from build123d import *

# Parameters (mm, degrees)
SKIZZE1_W                       = 89.6
SKIZZE1_H                       = 46
SKIZZE1_W_2                     = 86
SKIZZE1_H_2                     = 43
AUFSATZ_LINEAR_AUSTRAGEN1_DEPTH = 1
SKIZZE1_3_W                     = 89.6
SKIZZE1_3_H                     = 46
SKIZZE1_3_W_2                   = 86
SKIZZE1_3_H_2                   = 43
AUFSATZ_LINEAR_AUSTRAGEN2_DEPTH = 50
SKIZZE2_W                       = 5.5
SKIZZE2_H                       = 5.5
SKIZZE2_R                       = 1.45
AUFSATZ_LINEAR_AUSTRAGEN3_DEPTH = 15
SKIZZE3_W                       = 5.5
SKIZZE3_H                       = 5.5
AUFSATZ_LINEAR_AUSTRAGEN4_DEPTH = 0.5
FASE1_SIZE                      = 5.5
SKIZZE4_W                       = 4.158916141
SKIZZE4_H                       = 8.076735696
SCHNITT_LINEAR_AUSTRAGEN1_DEPTH = 10
SKIZZE5_W                       = 22.047742135
SKIZZE5_H                       = 8.787632461
SCHNITT_LINEAR_AUSTRAGEN2_DEPTH = 10
SKIZZE6_W                       = 19.779455906
SKIZZE6_H                       = 6.441932887
SCHNITT_LINEAR_AUSTRAGEN3_DEPTH = 10
SKIZZE9_W                       = 20
SKIZZE9_H                       = 6
AUFSATZ_LINEAR_AUSTRAGEN6_DEPTH = 10
SKIZZE10_R                      = 2.25
SCHNITT_LINEAR_AUSTRAGEN5_DEPTH = 10
SKIZZE11_W                      = 75
SKIZZE11_H                      = 0.1
SCHNITT_LINEAR_AUSTRAGEN6_DEPTH = 37.646803
SKIZZE12_W                      = 12
SKIZZE12_H                      = 4
AUFSATZ_LINEAR_AUSTRAGEN7_DEPTH = 20
SCHNITT_LINEAR_AUSTRAGEN7_REACH = 88.161
SKIZZE13_R                      = 2.25
SKIZZE14_R                      = 3.7
SCHNITT_LINEAR_AUSTRAGEN8_DEPTH = 2
SKIZZE15_W                      = 89.6
SKIZZE15_H                      = 4.2
AUFSATZ_LINEAR_AUSTRAGEN8_DEPTH = 20
FASE2_SIZE                      = 4.5
FASE3_SIZE                      = 5
FASE4_SIZE                      = 5
FASE5_SIZE                      = 6


# Some blends are built 0.0001 mm under size
with BuildPart() as part:
    # Skizze1 → Aufsatz-Linear austragen1 (new body)
    # profile 1 of 2: a face of its own
    with BuildSketch(Plane.XY):
        with Locations((0, -0.3)):
            Rectangle(SKIZZE1_W, SKIZZE1_H)
        Rectangle(SKIZZE1_W_2, SKIZZE1_H_2, mode=Mode.SUBTRACT)
    # profile 2 of 2: a face of its own
    with BuildSketch(Plane.XY):
        Rectangle(SKIZZE1_W_2, SKIZZE1_H_2)
    extrude(amount=AUFSATZ_LINEAR_AUSTRAGEN1_DEPTH)

    # Skizze1<3> → Aufsatz-Linear austragen2 (add)
    with BuildSketch(Plane.XY):
        with Locations((0, -0.3)):
            Rectangle(SKIZZE1_3_W, SKIZZE1_3_H)
        Rectangle(SKIZZE1_3_W_2, SKIZZE1_3_H_2, mode=Mode.SUBTRACT)
    extrude(amount=AUFSATZ_LINEAR_AUSTRAGEN2_DEPTH)

    # Skizze2 → Aufsatz-Linear austragen3 (add)
    # profile 1 of 4: a face of its own
    with BuildSketch(Plane.XY.offset(50)):
        with Locations((-40.25, 18.75)):
            Rectangle(SKIZZE2_W, SKIZZE2_H)
        with Locations((-40.5, 19)):
            Circle(SKIZZE2_R, mode=Mode.SUBTRACT)
    # profile 2 of 4: a face of its own
    with BuildSketch(Plane.XY.offset(50)):
        with Locations((-40.25, -18.75)):
            Rectangle(SKIZZE2_W, SKIZZE2_H)
        with Locations(Location((-40.5, -19, 0), (0, 0, 180))):
            Circle(SKIZZE2_R, mode=Mode.SUBTRACT)
    # profile 3 of 4: a face of its own
    with BuildSketch(Plane.XY.offset(50)):
        with Locations((40.25, -18.75)):
            Rectangle(SKIZZE2_W, SKIZZE2_H)
        with Locations((40.5, -19)):
            Circle(SKIZZE2_R, mode=Mode.SUBTRACT)
    # profile 4 of 4: a face of its own
    with BuildSketch(Plane.XY.offset(50)):
        with Locations((40.25, 18.75)):
            Rectangle(SKIZZE2_W, SKIZZE2_H)
        with Locations(Location((40.5, 19, 0), (0, 0, 180))):
            Circle(SKIZZE2_R, mode=Mode.SUBTRACT)
    extrude(amount=-AUFSATZ_LINEAR_AUSTRAGEN3_DEPTH)

    # Skizze3 → Aufsatz-Linear austragen4 (add)
    with BuildSketch(Plane(origin=(0, 0, 35), x_dir=(-1, 0, 0), z_dir=(0, 0, -1))):
        with Locations((-40.25, 18.75)):
            Rectangle(SKIZZE3_W, SKIZZE3_H)
        with Locations((-40.25, -18.75)):
            Rectangle(SKIZZE3_W, SKIZZE3_H)
        with Locations((40.25, -18.75)):
            Rectangle(SKIZZE3_W, SKIZZE3_H)
        with Locations((40.25, 18.75)):
            Rectangle(SKIZZE3_W, SKIZZE3_H)
    extrude(amount=AUFSATZ_LINEAR_AUSTRAGEN4_DEPTH)

    # Fase1
    fase1_edges = [part.edges().sort_by_distance(p)[0] for p in [
        (43, 18.75, 34.5),
        (40.25, 21.5, 34.5),
        (-40.25, -21.5, 34.5),
        (-43, -18.75, 34.5),
        (-43, 18.75, 34.5),
        (-40.25, 21.5, 34.5),
        (40.25, -21.5, 34.5),
        (43, -18.75, 34.5),
    ]]
    chamfer(fase1_edges, length=FASE1_SIZE - 0.0001)  # a hair under: the kernel refuses the full size

    # Skizze4 → Schnitt-Linear austragen1 (cut)
    with BuildSketch(Plane.ZY.offset(44.8)):
        with Locations((45.583621194, -0.3)):
            Rectangle(SKIZZE4_W, SKIZZE4_H)
    extrude(amount=-SCHNITT_LINEAR_AUSTRAGEN1_DEPTH, mode=Mode.SUBTRACT)

    # Skizze5 → Schnitt-Linear austragen2 (cut)
    with BuildSketch(Plane.XZ.offset(23.3)):
        with Locations((11.862553209, 7.95938084)):
            Rectangle(SKIZZE5_W, SKIZZE5_H)
    extrude(amount=-SCHNITT_LINEAR_AUSTRAGEN2_DEPTH, mode=Mode.SUBTRACT)

    # Skizze6 → Schnitt-Linear austragen3 (cut)
    with BuildSketch(Plane(origin=(0, 22.7, 0), x_dir=(1, 0, 0), z_dir=(0, 1, 0))):
        with Locations((0, -6.581515831)):
            Rectangle(SKIZZE6_W, SKIZZE6_H)
    extrude(amount=-SCHNITT_LINEAR_AUSTRAGEN3_DEPTH, mode=Mode.SUBTRACT)

    # Skizze9 → Aufsatz-Linear austragen6 (add)
    with BuildSketch(Plane(origin=(44.8, 0, 0), x_dir=(0, 0, -1), z_dir=(1, 0, 0))):
        with Locations((-40, -24.5)):
            Rectangle(SKIZZE9_W, SKIZZE9_H)
    extrude(amount=AUFSATZ_LINEAR_AUSTRAGEN6_DEPTH)

    # Skizze10 → Schnitt-Linear austragen5 (cut)
    with BuildSketch(Plane(origin=(0, -21.5, 0), x_dir=(1, 0, 0), z_dir=(0, 1, 0))):
        with Locations(Location((49.8, -40, 0), (0, 0, 180))):
            Circle(SKIZZE10_R)
        with Locations((-49.8, -40)):
            Circle(SKIZZE10_R)
    extrude(amount=-SCHNITT_LINEAR_AUSTRAGEN5_DEPTH, mode=Mode.SUBTRACT)

    # Skizze11 → Schnitt-Linear austragen6 (cut)
    with BuildSketch(Plane.XY.offset(50)):
        with Locations((0, -21.55)):
            Rectangle(SKIZZE11_W, SKIZZE11_H)
    extrude(amount=-SCHNITT_LINEAR_AUSTRAGEN6_DEPTH, mode=Mode.SUBTRACT)

    # Skizze12 → Aufsatz-Linear austragen7 (add)
    with BuildSketch(Plane.XY.offset(50)):
        with Locations((-50.8, -20.500000001)):
            Rectangle(SKIZZE12_W, SKIZZE12_H)
    extrude(amount=-AUFSATZ_LINEAR_AUSTRAGEN7_DEPTH)

    # Skizze13 → Schnitt-Linear austragen7 (cut, up to next)
    with BuildSketch(Plane(origin=(0, -18.500000001, 0), x_dir=(1, 0, 0), z_dir=(0, 1, 0)), mode=Mode.PRIVATE) as schnitt_linear_austragen7_sk1:
        with Locations(Location((-50.8, -40, 0), (0, 0, 180))):
            Circle(SKIZZE13_R)
    schnitt_linear_austragen7_tool1 = extrude(schnitt_linear_austragen7_sk1.sketch, amount=-SCHNITT_LINEAR_AUSTRAGEN7_REACH, mode=Mode.PRIVATE) & part.part
    add(schnitt_linear_austragen7_tool1.solids().sort_by_distance((-50.8, -18.5, 40))[0], mode=Mode.SUBTRACT)

    # Skizze14 → Schnitt-Linear austragen8 (cut)
    with BuildSketch(Plane(origin=(0, -18.500000001, 0), x_dir=(1, 0, 0), z_dir=(0, 1, 0))):
        with Locations(Location((-50.8, -40, 0), (0, 0, 180))):
            Circle(SKIZZE14_R)
    extrude(amount=-SCHNITT_LINEAR_AUSTRAGEN8_DEPTH, mode=Mode.SUBTRACT)

    # Skizze15 → Aufsatz-Linear austragen8 (add)
    with BuildSketch(Plane.XY.offset(50)):
        with Locations((0, -25.4)):
            Rectangle(SKIZZE15_W, SKIZZE15_H)
    extrude(amount=-AUFSATZ_LINEAR_AUSTRAGEN8_DEPTH)

    # Fase2
    # the kernel refuses this chamfer: 4.5 mm, written as the material it adds along each edge
    with BuildSketch(Plane(origin=(-44.8, -23.3, 30), x_dir=(0, 0.02749587661058602, -0.9996219169112969), z_dir=(1, 0, 0))) as fase2_piece_1_section:
        Polygon((FASE2_SIZE * 0.999621916911, -FASE2_SIZE * 0.0274958766106), (-FASE2_SIZE * 0.0274958766106, -FASE2_SIZE * 0.999621916911), (0, 0), align=None)
    fase2_piece_1 = extrude(amount=89.6, mode=Mode.PRIVATE)
    fase2_piece_1 = split(fase2_piece_1, bisect_by=Plane(origin=(0, -27.5, 28.499089477), z_dir=(0, 1, 0)), keep=Keep.TOP, mode=Mode.PRIVATE)
    add(fase2_piece_1)

    # Fase3
    fase3_edges = [part.edges().sort_by_distance(p)[0] for p in [
        (44.8, -24.5, 30),
    ]]
    chamfer(fase3_edges, length=FASE3_SIZE)

    # Fase4
    fase4_edges = [part.edges().sort_by_distance(p)[0] for p in [
        (54.8, -24.5, 30),
    ]]
    chamfer(fase4_edges, length=FASE4_SIZE - 0.0001)  # a hair under: the kernel refuses the full size

    # Fase5
    fase5_edges = [part.edges().sort_by_distance(p)[0] for p in [
        (-44.8, -20.500000001, 30),
    ]]
    chamfer(fase5_edges, length=FASE5_SIZE)
    fase5_2_edges = [part.edges().sort_by_distance(p)[0] for p in [
        (-56.8, -20.500000001, 30),
    ]]
    chamfer(fase5_2_edges, length=FASE5_SIZE - 0.0001)  # a hair under: the kernel refuses the full size


solid = part.part
CAD build for the part. Positions are in the model's coordinates, mm. A direction names the side the tool comes from. Give positions to 0.01 mm unless a question says otherwise; leave off trailing zeros. Order: outer loops, then holes, each group sorted by start corner. A loop starts at its lowest first (then second) coordinate and runs counter-clockwise, first axis right, second up. Notation, with made-up numbers: (80, 75) -> (105, 75) arc R21 ccw to (105, 104) -> close; hole circle Ø6 at (84, 81.5). An arc over 180 degrees is marked (long way). Return JSON: item names as keys, results as strings.
Q1. Saw through at D-D (z = 40). Count the separate pieces of the cut face and the enclosed holes in it, then the cut area to 3 significant figures.
Working result:
{"separate pieces": "3", "enclosed holes": "5", "area": "944 mm²"}
Q2. Saw through at A-A (z = 18.5). Write the cut outline in (x, y), then the cut area to 3 significant figures.
Working result:
{"outline": "(-44.8, -23.3) -> (44.8, -23.3) -> (44.8, 22.7) -> (-44.8, 22.7) -> close; hole (-43, -21.5) -> (-37.5, -21.5) -> (-37.5, -21.6) -> (37.5, -21.6) -> (37.5, -21.5) -> (43, -21.5) -> (43, 21.5) -> (-43, 21.5) -> close", "area": "416 mm²"}
Q3. Saw through at B-B (y = 1). Write the cut outline in (x, z), then the cut area to 3 significant figures.
Working result:
{"outline": "(-44.8, 0) -> (44.8, 0) -> (44.8, 50) -> (43, 50) -> (43, 1) -> (-43, 1) -> (-43, 43.5) -> (-44.8, 43.5) -> close; (-44.8, 47.66) -> (-43, 47.66) -> (-43, 50) -> (-44.8, 50) -> close", "area": "259 mm²"}
Q4. Saw through at C-C (y = -10.5). Write the cut outline in (x, z), then the cut area to 3 significant figures.
Working result:
{"outline": "(-44.8, 0) -> (44.8, 0) -> (44.8, 50) -> (43, 50) -> (43, 1) -> (-43, 1) -> (-43, 50) -> (-44.8, 50) -> close", "area": "266 mm²"}
Q5. Drill centre lines: line 1 (Y direction, x = -40.5, z = 41); line 2 (Y direction, x = -0.5, z = 14.5); line 3 (X direction, y = 8, z = 43.5). Where is each one in solid material? Low to high.
Working result:
{"line 1": "-27.5 to -20.45, -17.55 to -16, 16 to 17.55, 20.45 to 22.7", "line 2": "-23.3 to -21.6, 21.5 to 22.7", "line 3": "-44.8 to -43, 43 to 44.8"}
Q6. Mould opens along Z. For faces 5 (the face through (44.8, 0, 25)), 6 (the face through (39.1, 19.9, 30.6)), 7 (the face through (-40, 19, 35)) say: pulls with the +Z half, pulls with the -Z half, needs draft (parallel to the pull), parting line crosses it, or undercut.
Working result:
{"face 5": "needs draft", "face 6": "undercut", "face 7": "pulls with the +Z half"}
Q7. Which spindle directions (+Z, -Z, +X, -X, +Y, -Y) get a long thin tool onto all of the face, cutting with end or side? Do faces 1 (the face through (-1, -21.6, 31)), 2 (the face through (48.6, -21.5, 37.7)), 3 (the face through (0, -23.3, 13)), 4 (the face through (-41, 18, 31)). Say none if no direction does.
Working result:
{"face 1": "+Z", "face 2": "+Z, -Z, +X, +Y", "face 3": "-Z, +X, -X, -Y", "face 4": "none"}
Q8. Flat gauge pins, fed straight in: pin 1 (1.5 mm diameter, centred on y = -2, z = 29.5, fed in from -X); pin 2 (1 mm diameter, centred on y = 13, z = 8, fed in from +X); pin 3 (2 mm diameter, centred on x = -52.5, z = 38.5, fed in from +Y). Where does each tip first touch, or does it go through?
Working result:
{"pin 1": "x = -44.8", "pin 2": "x = 44.8", "pin 3": "y = -20.5"}
